The listing builds one solid part. Answer for the finished solid, in the listing's coordinates (mm). Face numbers are marked on the shaded views. A direction names the side the tool comes from. Round coordinates to 2 decimals unless told otherwise and drop trailing zeros. Write each loop counter-clockwise with the first axis right and the second up, starting at its lowest first coordinate (ties: lowest second). Pieces come first, ordered by that corner, then holes. Notation, with made-up numbers: (-7.75, -36) - (5.25, -36) arc R12 ccw to (5.25, -16) - close; hole circle Ø5 at (-30, 40.25). An arc over 180 degrees is marked (long way). Return JSON: item names as keys, results as strings. Group by question number.
(1) Find the intervals of material crossed by line 1 along Z through (x, y) = (8.89, 77.55); line 2 along Y through (x, z) = (9.25, -7.25); line 3 along Z through (x, y) = (8.89, 81.95), in increasing order. Write a range as [from, to].
(2) Section A-A, the plane x = 10 is taken. Write down the section's boundary in (y, z).
(3) Which of the six approach directions +Z, -Z, +X, -X, +Y, -Y give full straight-line access (tool end or side, diameter ignored) to the marked faces 1, 2 and 3?
(4) Section C-C, the plane z = -9 is taken. Write down the section's boundary in (x, y).
(5) Section B-B, the plane y = 64 is taken. Write down the section's boundary in (x, z), then the cut area to 3 significant figures.
(6) Each of these flat-tipped pins is pushed along its axis until it touches: pin 1 (2 mm diameter, centred on x = 9, z = -7.5, fed in from +Y); pin 2 (1.6 mm diameter, centred on x = 13.89, z = -3.81, fed in from -Y) (3 decimals); pin 3 (7.5 mm diameter, centred on x = 9.5, y = 52.5, fed in from +Z). Where does it stop, or does it pass through?
(7) Determine the mould class of the marked faces 4, 5 and 6 for opening direction Z: +Z half, -Z half, draft (parallel to the pull), parting line (faces both ways), or undercut.
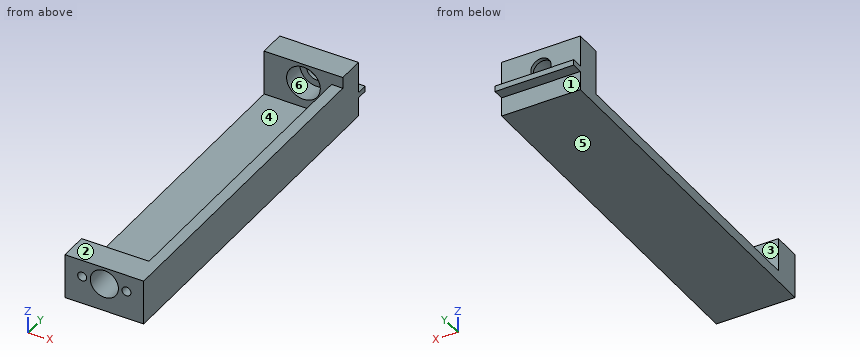
Autodesk Inventor part; units mm, degrees
ref_plane "YZ Plane" through (0, 0, 0) normal (1, 0, 0) x (0, 1, 0)
ref_plane "XZ Plane" through (0, 0, 0) normal (0, 1, 0) x (-1, 0, 0)
ref_plane "XY Plane" through (0, 0, 0) normal (0, 0, 1) x (1, 0, 0)
sketch "Sketch1" plane through (0, 0, 0) normal (0, 1, 0) x (-1, 0, 0)
  line L0 (0, 0) -> (-17.78, 0)
  line L1 (-17.78, 0) -> (-17.78, -10.16)
  line L2 (-17.78, -10.16) -> (0, -10.16)
  line L3 (0, -10.16) -> (0, 0)
  dimension "d0" = 17.78
  dimension "d1" = 10.16
extrude "Extrusion1" add sketch "Sketch1" along normal blind 82.296
sketch "Sketch2" plane through (0, 0, 0) normal (0, -1, 0) x (1, 0, 0)
  line L0 (0, 0) -> (0, -5.08)
  line L1 (0, -10.16) -> (0, 0)
  line L2 (0, 0) -> (17.78, 0)
  line L3 (8.89, 0) -> (8.89, -3.81)
  circle A0 centre (8.89, -3.81) radius 3.175
  line L4 (8.89, -3.81) -> (11.8809, -3.81)
  line L5 (8.89, -3.81) -> (3.8862, -3.81)
  line L6 (8.89, -3.81) -> (13.8938, -3.81)
  circle A1 centre (13.8938, -3.81) radius 1.016
  circle A2 centre (3.8862, -3.81) radius 1.016
  dimension "d5" = 6.35
  dimension "d6" = 5.0038
  dimension "d7" = 5.0038
  dimension "d8" = 2.032
  dimension "d9" = 2.032
  dimension "d20" = 3.81
extrude "Extrusion2" cut sketch "Sketch2" against normal blind 50.8 contours A0 L6 L4 L3 | L3 L5 A0 | L4 L6 A0 L5
sketch "Sketch3" plane through (0, 0, 0) normal (0, 0, 1) x (1, 0, 0)
  line L0 (0, 0) -> (0, 82.296)
  line L1 (0, 0) -> (0, 6.35)
  line L2 (0, 6.35) -> (15.24, 6.35)
  line L3 (15.24, 6.35) -> (-24.1406, 6.35)
  line L4 (-24.1406, 6.35) -> (-24.1406, 76.3224)
  line L5 (-24.1406, 76.3224) -> (15.24, 76.3224)
  line L6 (15.24, 76.3224) -> (15.24, 6.35)
  point P0 (0, 76.3224)
  dimension "d12" = 6.35
  dimension "d13" = 15.24
extrude "Extrusion3" cut sketch "Sketch3" against normal blind 7.62 contours L0 L5 L6 L2
extrude "Extrusion4" cut sketch "Sketch2" against normal blind 4.445 contours A1 | A2
thread "Thread1"
sketch "Sketch4" plane through (0, 82.296, 0) normal (0, 1, 0) x (1, 0, 0)
  circle A0 centre (8.89, 3.81) radius 3.175
  line L0 (8.89, 0) -> (8.89, 3.81)
  circle A1 centre (8.89, 3.81) radius 2.286
  line L1 (8.89, 3.81) -> (8.89, 1.9304)
  circle A2 centre (8.89, 1.9304) radius 2.286
  point P0 (0, 0)
  dimension "d21" = 4.572
  dimension "d28" = 1.8796
  dimension "d29" = 4.572
sketch "Sketch5" plane through (0, 82.296, 0) normal (0, 1, 0) x (1, 0, 0)
  circle A0 centre (8.89, 3.81) radius 2.286
  line L0 (8.89, 3.81) -> (8.89, 6.477)
  line L1 (8.89, 6.477) -> (0, 6.477)
  line L2 (0, 10.16) -> (0, 0)
  line L3 (8.89, 6.477) -> (17.78, 6.477)
  line L4 (17.78, 0) -> (17.78, 10.16)
  line L5 (17.78, 6.477) -> (17.78, 7.747)
  line L6 (17.78, 7.747) -> (0, 7.747)
  line L7 (0, 6.477) -> (0, 7.747)
  line L8 (8.89, 3.81) -> (8.89, 1.9304)
  line L9 (8.89, 6.477) -> (8.89, 4.5974)
  line L10 (8.89, 4.5974) -> (0, 4.5974)
  line L11 (8.89, 4.5974) -> (17.78, 4.5974)
  line L12 (17.78, 5.8674) -> (0, 5.8674)
  line L13 (17.78, 4.5974) -> (17.78, 5.8674)
  line L14 (0, 4.5974) -> (0, 5.8674)
  point P0 (0, 5.8674)
  point P1 (0, 4.5974)
  dimension "d24" = 2.667
  dimension "d25" = 1.27
  dimension "d35" = 1.8796
  dimension "d36" = 1.8796
  dimension "d37" = 1.27
sketch "Sketch6" plane through (0, 82.296, 0) normal (0, 1, 0) x (1, 0, 0)
  line L0 (0, 0) -> (17.78, 0)
  line L1 (0, 0) -> (17.78, 0)
  line L2 (17.78, 0) -> (17.78, -2.54)
  line L3 (17.78, -2.54) -> (0, -2.54)
  line L4 (0, -2.54) -> (0, 0)
  dimension "d30" = 2.54
extrude "Extrusion7" add sketch "Sketch6" against normal blind 5.9736
extrude "Extrusion8" cut sketch "Sketch4" against normal blind 25.4 contours A2 A1 L0 A0 | A0 A2 | A0 L0 A1 A2 | A2 A1 picked at (9.0633, 2.4414)
extrude "Extrusion9" add sketch "Sketch5" along normal blind 2.54 contours L11 L0 L12 A0 | A0 L12 L4 L11 | L10 L2 L12 A0 | A0 L12 L0 L10
sketch "Sketch8" plane through (0, 76.3224, -7.62) normal (0, -1, 0) x (1, 0, 0)
  circle A0 centre (8.89, 5.6896) radius 2.286
  circle A1 centre (8.89, 5.6896) radius 2.286
  circle A2 centre (8.89, 5.6896) radius 3.81
  point P0 (0, 7.62)
  point P1 (10.1145, 7.62)
  point P2 (7.6655, 7.62)
  dimension "d41" = 7.62
extrude "Extrusion10" cut sketch "Sketch8" against normal blind 5.08
properties part number "IDA12toPolarisAdapter"
Working result:
{
 "1": {"line 1": "z = [-10.16, -5.74], [1.88, 2.54]", "line 2": "y = [0, 6.35], [76.32, 82.3]", "line 3": "z = [-10.16, -4.22], [0.36, 2.54]"},
 "2": {"outline": "(0, -10.16) - (82.3, -10.16) - (82.3, -5.87) - (84.84, -5.87) - (84.84, -4.6) - (82.3, -4.6) - (82.3, -3.93) - (81.4, -3.93) - (81.4, -5.58) - (76.32, -5.58) - (76.32, -7.62) - (6.35, -7.62) - (6.35, -6.78) - (0, -6.78) - close; (0, -0.84) - (6.35, -0.84) - (6.35, 0) - (0, 0) - close; (76.32, 1.71) - (81.4, 1.71) - (81.4, 0.07) - (82.3, 0.07) - (82.3, 2.54) - (76.32, 2.54) - close"},
 "3": {"face 1": "-Z, +X, -X, +Y", "face 2": "+Z, +X, -X, -Y", "face 3": "+Z, -X"},
 "4": {"outline": "(0, 0) - (17.78, 0) - (17.78, 82.3) - (0, 82.3) - close"},
 "5": {"outline": "(0, -10.16) - (17.78, -10.16) - (17.78, 0) - (15.24, 0) - (15.24, -7.62) - (0, -7.62) - close", "area": "64.5 mm^2"},
 "6": {"pin 1": "stops at y = 82.3", "pin 2": "stops at y = 4.445", "pin 3": "stops at z = -7.62"},
 "7": {"face 4": "+Z half", "face 5": "-Z half", "face 6": "undercut"}
}
